Work out the finished part from the listing and answer in its coordinate system (mm). A direction names the side the tool comes from. Give positions to 0.01 mm unless a question says otherwise; leave off trailing zeros. Order: outer loops, then holes, each group sorted by start corner. A loop starts at its lowest first (then second) coordinate and runs counter-clockwise, first axis right, second up.
```python
from build123d import *

# Parameters (mm, degrees)
SKETCH1_R                      = 2.65
BOSS_EXTRUDE1_DEPTH            = 11.53
CUT_EXTRUDE1_START             = -10.785
CUT_EXTRUDE1_DEPTH             = 10.785
CUT_EXTRUDE3_REACH             = 27.381
SKETCH10_R                     = 0.625
CUT_EXTRUDE3_DIRECTION_2_REACH = 27.381
CUT_EXTRUDE2_REACH             = 33.272
SKETCH5_R                      = 0.625
BOSS_EXTRUDE2_DEPTH            = 3.5
BOSS_EXTRUDE3_DEPTH            = 2


with BuildPart() as part:
    # Sketch1 → Boss-Extrude1 (new body)
    with BuildSketch(Plane(origin=(0, 0, 0), x_dir=(1, 0, 0), z_dir=(0, 1, 0))):
        with BuildLine():
            Line((-11, -13), (11, -13))
            ThreePointArc((11, -13), (12.414213562, -12.414213562), (13, -11))
            Line((13, -11), (13, 11))
            ThreePointArc((13, 11), (12.414213562, 12.414213562), (11, 13))
            Line((11, 13), (-11, 13))
            ThreePointArc((-11, 13), (-12.414213562, 12.414213562), (-13, 11))
            Line((-13, 11), (-13, -11))
            ThreePointArc((-13, -11), (-12.414213562, -12.414213562), (-11, -13))
        make_face()
        with Locations(Location((5, 0, 0), (0, 0, 270))):
            Circle(SKETCH1_R, mode=Mode.SUBTRACT)
        with Locations(Location((-5, 0, 0), (0, 0, 270))):
            Circle(SKETCH1_R, mode=Mode.SUBTRACT)
    extrude(amount=BOSS_EXTRUDE1_DEPTH)

    # Sketch2 → Cut-Extrude1 (cut)
    with BuildSketch(Plane(origin=(0, 11.53, 0), x_dir=(1, 0, 0), z_dir=(0, 1, 0)).offset(CUT_EXTRUDE1_START)):
        with BuildLine():
            Line((4.5, 3.65), (4.5, 2.602402736))
            ThreePointArc((4.5, 2.602402736), (5, 2.65), (5.5, 2.602402736))
            Line((5.5, 2.602402736), (5.5, 3.65))
            Line((5.5, 3.65), (4.5, 3.65))
        make_face()
        with BuildLine():
            ThreePointArc((7.65, 0), (7.638073848, -0.251130195), (7.602402736, -0.5))
            Line((7.602402736, -0.5), (8.65, -0.5))
            Line((8.65, -0.5), (8.65, 0.5))
            Line((8.65, 0.5), (7.602402736, 0.5))
            ThreePointArc((7.602402736, 0.5), (7.638073848, 0.251130195), (7.65, 0))
        make_face()
        with BuildLine():
            Line((4.5, -2.602402736), (4.5, -3.65))
            Line((4.5, -3.65), (5.5, -3.65))
            Line((5.5, -3.65), (5.5, -2.602402736))
            ThreePointArc((5.5, -2.602402736), (5, -2.65), (4.5, -2.602402736))
        make_face()
        with BuildLine():
            Line((1.35, -0.5), (2.397597264, -0.5))
            ThreePointArc((2.397597264, -0.5), (2.35, 0), (2.397597264, 0.5))
            Line((2.397597264, 0.5), (1.35, 0.5))
            Line((1.35, 0.5), (1.35, -0.5))
        make_face()
        with BuildLine():
            ThreePointArc((-2.35, 0), (-2.361926152, -0.251130195), (-2.397597264, -0.5))
            Line((-2.397597264, -0.5), (-1.35, -0.5))
            Line((-1.35, -0.5), (-1.35, 0.5))
            Line((-1.35, 0.5), (-2.397597264, 0.5))
            ThreePointArc((-2.397597264, 0.5), (-2.361926152, 0.251130195), (-2.35, 0))
        make_face()
        with BuildLine():
            Line((-5.5, 3.65), (-5.5, 2.602402736))
            ThreePointArc((-5.5, 2.602402736), (-5, 2.65), (-4.5, 2.602402736))
            Line((-4.5, 2.602402736), (-4.5, 3.65))
            Line((-4.5, 3.65), (-5.5, 3.65))
        make_face()
        with BuildLine():
            Line((-8.65, 0.5), (-8.65, -0.5))
            Line((-8.65, -0.5), (-7.602402736, -0.5))
            ThreePointArc((-7.602402736, -0.5), (-7.65, 0), (-7.602402736, 0.5))
            Line((-7.602402736, 0.5), (-8.65, 0.5))
        make_face()
        with BuildLine():
            ThreePointArc((-4.5, -2.602402736), (-5, -2.65), (-5.5, -2.602402736))
            Line((-5.5, -2.602402736), (-5.5, -3.65))
            Line((-5.5, -3.65), (-4.5, -3.65))
            Line((-4.5, -3.65), (-4.5, -2.602402736))
        make_face()
    extrude(amount=CUT_EXTRUDE1_DEPTH, mode=Mode.SUBTRACT)

    # Sketch3 → Revolve1 (revolve)
    with BuildSketch(Plane(origin=(0, 0, 0), x_dir=(0, 0, -1), z_dir=(1, 0, 0)), mode=Mode.PRIVATE) as revolve1_sk:
        Polygon((-13, 0.3), (-16, 0.3), (-16, 0), (-18.5, 0.5), (-18.5, 0.75), (-13, 0.75), align=None)
    revolve(revolve1_sk.sketch.rotate(Axis((0, 1.375, 13), (0, 0, 1)), 180), axis=Axis((0, 1.375, 13), (0, 0, 1)))

    # Sketch10 → Cut-Extrude3 (cut, up to next)
    with BuildSketch(Plane(origin=(0, 0, 0), x_dir=(0, 0, -1), z_dir=(1, 0, 0)), mode=Mode.PRIVATE) as cut_extrude3_sk1:
        with Locations(Location((0, 1.375, 0), (0, 0, 143.130102406))):
            Circle(SKETCH10_R)
    cut_extrude3_tool1 = extrude(cut_extrude3_sk1.sketch, amount=-CUT_EXTRUDE3_REACH, mode=Mode.PRIVATE) & part.part
    add(cut_extrude3_tool1.solids().sort_by_distance((0, 1.375, 0))[0], mode=Mode.SUBTRACT)

    # Sketch10 → Cut-Extrude3 direction 2 (cut, up to next)
    with BuildSketch(Plane(origin=(0, 0, 0), x_dir=(0, 0, -1), z_dir=(1, 0, 0)), mode=Mode.PRIVATE) as cut_extrude3_direction_2_sk1:
        with Locations(Location((0, 1.375, 0), (0, 0, 143.130102406))):
            Circle(SKETCH10_R)
    cut_extrude3_direction_2_tool1 = extrude(cut_extrude3_direction_2_sk1.sketch, amount=CUT_EXTRUDE3_DIRECTION_2_REACH, mode=Mode.PRIVATE) & part.part
    add(cut_extrude3_direction_2_tool1.solids().sort_by_distance((0, 1.375, 0))[0], mode=Mode.SUBTRACT)

    # Sketch5 → Cut-Extrude2 (cut, up to next)
    with BuildSketch(Plane.XY.offset(13), mode=Mode.PRIVATE) as cut_extrude2_sk1:
        with Locations(Location((0, 1.375, 0), (0, 0, 90))):
            Circle(SKETCH5_R)
    cut_extrude2_tool1 = extrude(cut_extrude2_sk1.sketch, amount=-CUT_EXTRUDE2_REACH, mode=Mode.PRIVATE) & part.part
    add(cut_extrude2_tool1.solids().sort_by_distance((0, 1.375, 13))[0], mode=Mode.SUBTRACT)

    # Sketch6 → Boss-Extrude2 (add)
    with BuildSketch(Plane(origin=(0, 11.53, 0), x_dir=(1, 0, 0), z_dir=(0, 1, 0))):
        with BuildLine():
            Line((-11, -13), (11, -13))
            ThreePointArc((11, -13), (12.414213562, -12.414213562), (13, -11))
            Line((13, -11), (13, 11))
            ThreePointArc((13, 11), (12.414213562, 12.414213562), (11, 13))
            Line((11, 13), (-11, 13))
            ThreePointArc((-11, 13), (-12.414213562, 12.414213562), (-13, 11))
            Line((-13, 11), (-13, -11))
            ThreePointArc((-13, -11), (-12.414213562, -12.414213562), (-11, -13))
        make_face()
        with BuildLine():
            Line((-8, -10), (8, -10))
            ThreePointArc((8, -10), (9.414213562, -9.414213562), (10, -8))
            Line((10, -8), (10, 8))
            ThreePointArc((10, 8), (9.414213562, 9.414213562), (8, 10))
            Line((8, 10), (-8, 10))
            ThreePointArc((-8, 10), (-9.414213562, 9.414213562), (-10, 8))
            Line((-10, 8), (-10, -8))
            ThreePointArc((-10, -8), (-9.414213562, -9.414213562), (-8, -10))
        make_face(mode=Mode.SUBTRACT)
    extrude(amount=BOSS_EXTRUDE2_DEPTH)

    # Sketch8 → Boss-Extrude3 (add)
    with BuildSketch(Plane(origin=(0, 15.03, 0), x_dir=(1, 0, 0), z_dir=(0, 1, 0))):
        with BuildLine():
            Line((-11, -13), (11, -13))
            ThreePointArc((11, -13), (12.414213562, -12.414213562), (13, -11))
            Line((13, -11), (13, 11))
            ThreePointArc((13, 11), (12.414213562, 12.414213562), (11, 13))
            Line((11, 13), (-11, 13))
            ThreePointArc((-11, 13), (-12.414213562, 12.414213562), (-13, 11))
            Line((-13, 11), (-13, -11))
            ThreePointArc((-13, -11), (-12.414213562, -12.414213562), (-11, -13))
        make_face()
        with BuildLine():
            Line((-10, -12), (10, -12))
            ThreePointArc((10, -12), (11.414213562, -11.414213562), (12, -10))
            Line((12, -10), (12, 10))
            ThreePointArc((12, 10), (11.414213562, 11.414213562), (10, 12))
            Line((10, 12), (-10, 12))
            ThreePointArc((-10, 12), (-11.414213562, 11.414213562), (-12, 10))
            Line((-12, 10), (-12, -10))
            ThreePointArc((-12, -10), (-11.414213562, -11.414213562), (-10, -12))
        make_face(mode=Mode.SUBTRACT)
    extrude(amount=BOSS_EXTRUDE3_DEPTH)


solid = part.part
```
1. Given P1, Ø1.1, axis at x = 5, z = 3.5, coming from the +Y side; P2, Ø5, axis at x = -5, y = 14, coming from the +Z side; P3, Ø4, axis at x = 2, z = 9, coming from the +Y side, each flat-ended and moving along its own axis, determine where each tip first touches the part or whether it passes through.
Findings below:
P1: stops at y = 11.53
P2: stops at z = 13
P3: stops at y = 15.03
2. The part is cut by section B-B (z = -5.5). Write down the section's boundary in (x, y).
Findings below:
outline: (-13, 0) - (13, 0) - (13, 17.03) - (12, 17.03) - (12, 15.03) - (10, 15.03) - (10, 11.53) - (-10, 11.53) - (-10, 15.03) - (-12, 15.03) - (-12, 17.03) - (-13, 17.03) - close
3. Straight lines are drawn through the part: probe 1 along X at (y, z) = (6.5, -3.5); probe 2 along X at (y, z) = (7, 0); probe 3 along Z at (x, y) = (2.25, 1). For each, find the intervals that lie inside material, in ascending order.
Findings below:
probe 1: x = -13 to -5.5, -4.5 to 4.5, 5.5 to 13
probe 2: x = -13 to -8.65, -1.35 to 1.35, 8.65 to 13
probe 3: z = -13 to -0.5, 0.5 to 13
4. The part is cut by section C-C (y = 4.5). State how many separate pieces and enclosed holes the cut face has, then the cut area to 3 significant figures.
Findings below:
separate pieces: 1
enclosed holes: 2
area: 620 mm2
5. The mould has two halves that part along Z. Classify faces 1 (the face through (12.4, 8.4, 12.43)), 2 (the face through (-1, 17.03, 12.5)), 3 (the face through (-9.4, 13.26, -9.43)): pulls with the +Z half, pulls with the -Z half, needs draft (parallel to the pull), parting line crosses it, or undercut.
Findings below:
face 1: pulls with the +Z half
face 2: needs draft
face 3: undercut
6. The part is cut by section D-D (z = 12.5). Write down the section's boundary in (x, y) (3 decimals).
Findings below:
outline: (-12.323, 0) - (12.323, 0) - (12.323, 17.03) - (-12.323, 17.03) - close; hole circle Ø1.25 at (0, 1.375)
7. The part is cut by section A-A (x = 5). Write down the section's boundary in (y, z) (3 decimals).
Findings below:
outline: (0, -13) - (17.03, -13) - (17.03, -12) - (15.03, -12) - (15.03, -10) - (11.53, -10) - (11.53, -3.65) - (0.745, -3.65) - (0.745, -2.65) - (0, -2.65) - close; (0, 2.65) - (0.745, 2.65) - (0.745, 3.65) - (11.53, 3.65) - (11.53, 10) - (15.03, 10) - (15.03, 12) - (17.03, 12) - (17.03, 13) - (0, 13) - close
8. Which of the six approach directions +Z, -Z, +X, -X, +Y, -Y give full straight-line access (tool end or side, diameter ignored) to faces 4 (the face through (12.43, 8.4, -12.4)), 5 (the face through (-10, 13, 0)), 6 (the face through (0, 0.3, 14.5))?
Findings below:
face 4: -Z, +X, +Y, -Y
face 5: +Y
face 6: none
